Check sheet for the drawn part. Datum: minimum x, y, z corner. Units: mm. A direction names the side the tool comes from. Round coordinates to 2 decimals unless told otherwise and drop trailing zeros. Order: outer loops, then holes, each group sorted by start corner. A loop starts at its lowest first (then second) coordinate and runs counter-clockwise, first axis right, second up. Notation, with made-up numbers: M 54,-29.5 L 64,-29.5 A17 ccw 64,-13.5 Z; hole C 84.25,49.5 d3. An arc over 180 degrees is marked long. Write item = value, one per line. Start each with the question number.
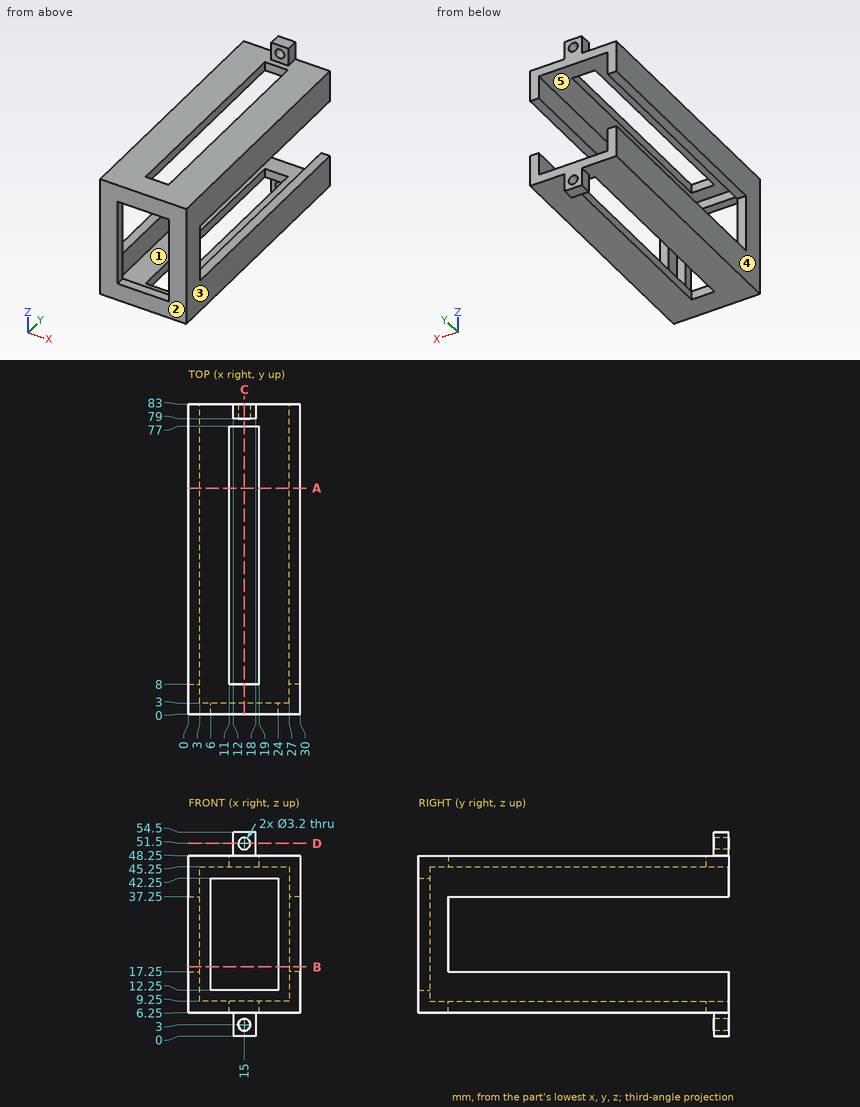
1) Gauge pin test, flat ends, axial feed: P1, Ø2.5, axis at x = 15, z = 3, coming from the +Y side; P2, Ø8, axis at x = 6, y = 36, coming from the -Z side; P3, Ø4, axis at x = 15, z = 51.5, coming from the -Y side; P4, Ø6, axis at x = 9, y = 59.5, coming from the +Z side. Record the tip position at first contact, or that the pin passes through.
2) Cross-section at D-D, the plane z = 51.5. Enter the section's corners in (x, y), then the cut area to 3 significant figures.
3) Scan lines: probe 1 along Z at (x, y) = (15, 80.4); probe 2 along X at (y, z) = (80, 3); probe 3 along X at (y, z) = (49, 40). Record each from-to range of solid material in increasing order.
4) Access from +Z, -Z, +X, -X, +Y, -Y to the whole of each face (thin tool, end or side, straight path). Record for the marked faces 4 and 5.
5) Release check for a two-part mould opening along X. For the marked faces 1, 2 and 3 record: pulls with the +X half, pulls with the -X half, needs draft (parallel to the pull), parting line crosses it, or undercut.
6) Cross-section at B-B, the plane z = 18.5. Enter the section's corners in (x, y), then the cut area to 3 significant figures.
7) Cross-section at A-A, the plane y = 60.5. Enter the section's corners in (x, z).
8) Cross-section at C-C, the plane x = 15. Give the number of separate pieces and of enclosed holes in the cut face, then the cut area to 3 significant figures.
Geometry results:
q1.P1 = through
q1.P2 = 6.25
q1.P3 = 79
q1.P4 = 48.25
q2.outline = M 12,79 L 13.4,79 L 13.4,83 L 12,83 Z; M 16.6,79 L 18,79 L 18,83 L 16.6,83 Z
q2.area = 11.2 mm^2
q3.probe_1 = 0 to 1.4, 4.6 to 9.25, 45.25 to 49.9, 53.1 to 54.5
q3.probe_2 = 12 to 13.4, 16.6 to 18
q3.probe_3 = 0 to 3, 27 to 30
q4.face_4 = +Z, -Z, -X, +Y, -Y
q4.face_5 = +Y
q5.face_1 = undercut
q5.face_2 = needs draft
q5.face_3 = pulls with the +X half
q6.outline = M 0,0 L 6,0 L 6,3 L 3,3 L 3,8 L 0,8 Z; M 24,0 L 30,0 L 30,8 L 27,8 L 27,3 L 24,3 Z
q6.area = 66.0 mm^2
q7.outline = M 0,6.25 L 11,6.25 L 11,9.25 L 3,9.25 L 3,17.25 L 0,17.25 Z; M 0,37.25 L 3,37.25 L 3,45.25 L 11,45.25 L 11,48.25 L 0,48.25 Z; M 19,6.25 L 30,6.25 L 30,17.25 L 27,17.25 L 27,9.25 L 19,9.25 Z; M 19,45.25 L 27,45.25 L 27,37.25 L 30,37.25 L 30,48.25 L 19,48.25 Z
q8.separate_pieces = 6
q8.enclosed_holes = 0
q8.area = 126 mm^2
